from build123d import *

# Parameters (mm, degrees)
BOSS_EXTRUDE3_DEPTH = 3


with BuildPart() as part:
    # Sketch4 → Boss-Extrude3 (new body)
    with BuildSketch(Plane(origin=(0, 0, 0), x_dir=(1, 0, 0), z_dir=(0, 1, 0))):
        with BuildLine():
            ThreePointArc((-3.047220201, 23.891690771), (-18.047220201, 8.891690771), (-3.047220201, -6.108309229))
            Line((-3.047220201, -6.108309229), (6.952779799, -6.108309229))
            Line((6.952779799, -6.108309229), (6.952779799, 23.891690771))
            Line((6.952779799, 23.891690771), (-3.047220201, 23.891690771))
        make_face()
        with BuildLine():
            Line((-7.047220201, 11.891690771), (0.952779799, 11.891690771))
            ThreePointArc((0.952779799, 11.891690771), (-3.047220201, 3.891690771), (-7.047220201, 11.891690771))
        make_face(mode=Mode.SUBTRACT)
    extrude(amount=BOSS_EXTRUDE3_DEPTH)


solid = part.part
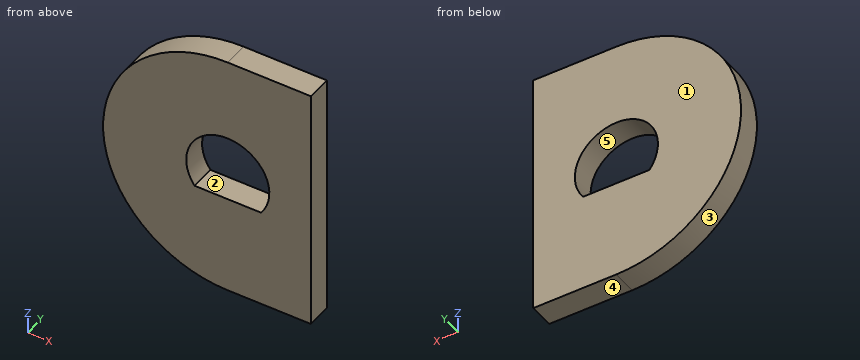
Check sheet for the modelled part. Datum: model origin and axes. Units: mm. Face numbers are marked on the shaded views. A direction names the side the tool comes from. Round coordinates to 2 decimals unless told otherwise and drop trailing zeros. Order: outer loops, then holes, each group sorted by start corner. A loop starts at its lowest first (then second) coordinate and runs counter-clockwise, first axis right, second up. Notation, with made-up numbers: M -20.75,71.5 L 12.25,71.5 A22 ccw 12.25,82.5 Z; hole C 20,-13.5 d6. An arc over 180 degrees is marked long. One line per item, written item: value. Start each with the question number.
1. Scan lines: line 1 along Z through (x, y) = (-4.25, 0.9); line 2 along X through (y, z) = (1.95, -7.25); line 3 along Z through (x, y) = (-4, 0.45). Record each from-to range of solid material in increasing order.
2. Access from +Z, -Z, +X, -X, +Y, -Y to the whole of each face (thin tool, end or side, straight path). Record for the marked faces 1 and 2.
3. Section check A-A on y = 0.95. Enter the section's corners in (x, z), and give its area (3 significant figures).
4. Gauge pin test, flat end, axial feed: P1, Ø1, axis at x = -9.5, y = 2.5, coming from the +Z side. Record the tip position at first contact, or that the pin passes through.
5. Section check D-D on z = -0.75. Enter the section's corners in (x, y), and give its area (3 significant figures).
6. Section check C-C on x = 1.5. Enter the section's corners in (y, z), and give its area (3 significant figures).
7. Section check B-B on x = -5. Enter the section's corners in (y, z), and give its area (3 significant figures).
8. Release check for a two-part mould opening along Z. For the marked faces 3, 4 and 5 record: released by +Z, released by -Z, zero draft, split by the parting line, or undercut.
Results found:
1. line 1: -23.84 to -11.89, -4.04 to 6.06
1. line 2: -17.96 to -7.77, 1.68 to 6.95
1. line 3: -23.86 to -11.89, -3.98 to 6.08
2. face 1: +Z, -Z, +X, -X, +Y
2. face 2: +Y, -Y
3. outline: M -3.05,-23.89 L 6.95,-23.89 L 6.95,6.11 L -3.05,6.11 A15 ccw Z; hole M -7.05,-11.89 L 0.95,-11.89 A5 ccw long Z
3. area: 586 mm^2
4. P1: z = 4.88
5. outline: M -15.65,0 L 6.95,0 L 6.95,3 L -15.65,3 Z
5. area: 67.8 mm^2
6. outline: M 0,-23.89 L 3,-23.89 L 3,-10.97 L 0,-10.97 Z; M 0,-6.81 L 3,-6.81 L 3,6.11 L 0,6.11 Z
6. area: 77.5 mm^2
7. outline: M 0,-23.76 L 3,-23.76 L 3,-11.89 L 0,-11.89 Z; M 0,-4.29 L 3,-4.29 L 3,5.98 L 0,5.98 Z
7. area: 66.4 mm^2
8. face 3: split by the parting line
8. face 4: released by -Z
8. face 5: undercut
